Verification items for the finished model (mm, model axes). Face numbers are marked on the shaded views. A direction names the side the tool comes from. Give positions to 0.01 mm unless a question says otherwise; leave off trailing zeros. Order: outer loops, then holes, each group sorted by start corner. A loop starts at its lowest first (then second) coordinate and runs counter-clockwise, first axis right, second up. Notation, with made-up numbers: (-18, 22) -> (-8, 22) arc R22 ccw to (-8, 42) -> close; hole circle Ø1 at (-38.5, 39.5). An arc over 180 degrees is marked (long way). Return JSON: item names as keys, results as strings. Group by question number.
(1) Thickness scan on line 1 along X through (y, z) = (-0.25, -9); line 2 along Z through (x, y) = (1.25, 3.5); line 3 along Z through (x, y) = (-1.75, 7). Record the ranges inside material, lowest first.
(2) Cross-section at B-B on z = -14. Enter the section's corners in (x, y), then the cut area to 3 significant figures.
(3) Cross-section at C-C on y = -3.75. Enter the section's corners in (x, z), then the cut area to 3 significant figures.
(4) Depth check by flat-ended pin: pin 1 Ø2 at (x, y) = (0.5, -4) entering from -Z; pin 2 Ø10 at (x, y) = (1.5, 4) entering from -Z; pin 3 Ø5 at (y, z) = (6.5, -12.5) entering from -X; pin 4 Ø0.6 at (x, z) = (1.5, -21) entering from +Y. Enter the tip coordinate at first touch or a pass-through.
(5) Tool access check on the marked faces 1 and 2. Record the directions out of +Z, -Z, +X, -X, +Y, -Y that give a thin tool (end or side, any length) a straight path to the whole face; none if there is none.
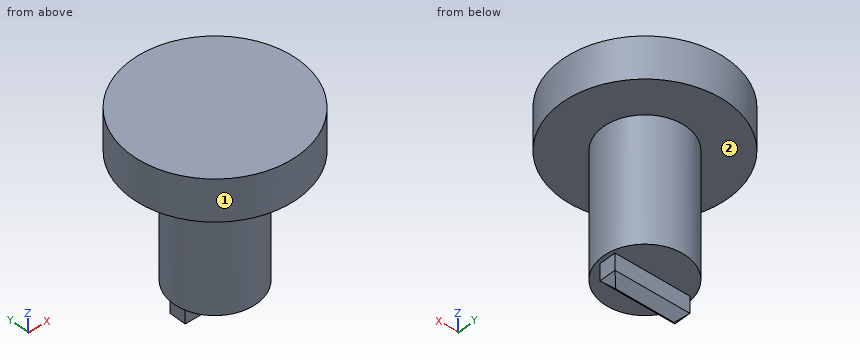
from build123d import *

# Parameters (mm, degrees)
F0_R     = 10
F1_DEPTH = 5
F2_R     = 5
F3_DEPTH = 15
F4_W     = 9
F4_H     = 2
F5_DEPTH = 3
F6_SIZE  = 0.99999


# Not quite as in the source:
# - a fillet or chamfer is up to 0.001 mm smaller than in the source, because OpenCascade refuses the exact size


with BuildPart() as f1:
    # F0 (on Top) → F1 (new body)
    with BuildSketch(Plane.XY):
        Circle(F0_R)
    extrude(amount=-F1_DEPTH)

    # F2 (on face) → F3 (join)
    with BuildSketch(Plane(origin=(0, 0, -5), x_dir=(1, 0, 0), z_dir=(0, 0, -1))):
        Circle(F2_R)
    extrude(amount=F3_DEPTH)

    # F4 (on face) → F5 (join)
    with BuildSketch(Plane(origin=(0, 0, -20), x_dir=(1, 0, 0), z_dir=(0, 0, -1))):
        Rectangle(F4_W, F4_H)
    extrude(amount=F5_DEPTH)

    # F6 (size 1 in the source; OpenCascade refuses exactly that, so slightly less here)
    f6_edges = [f1.edges().sort_by_distance(p)[0] for p in [
        (0, -1, -23),
        (-4.5, 0, -23),
        (0, 1, -23),
        (4.5, 0, -23),
    ]]
    chamfer(f6_edges, length=F6_SIZE)


solid = f1.part
Verdict:
{
 "1": {"line 1": "-4.99 to 4.99", "line 2": "-20 to 0", "line 3": "-5 to 0"},
 "2": {"outline": "circle Ø10 at (0, 0)", "area": "78.5 mm²"},
 "3": {"outline": "(-9.27, -5) -> (-3.31, -5) -> (-3.31, -20) -> (3.31, -20) -> (3.31, -5) -> (9.27, -5) -> (9.27, 0) -> (-9.27, 0) -> close", "area": "192 mm²"},
 "4": {"pin 1": "z = -20", "pin 2": "z = -23", "pin 3": "x = -3", "pin 4": "y = 1"},
 "5": {"face 1": "+Z, -Z", "face 2": "-Z"}
}
